Job drawing, mm, ordinate dimensions from the low corner. One solid piece. A direction names the side the tool comes from. Coordinates: 2 decimals unless noted, no trailing zeros. Loops run counter-clockwise (first coordinate to the right, second up) from the corner with the lowest first, then second, coordinate; pieces in that order, holes last. Notation, with made-up numbers: (-18.5, 62.5) -> (7.5, 62.5) arc R13 ccw to (7.5, 80.5) -> close; hole circle Ø4 at (33.5, 89). An arc over 180 degrees is marked (long way). Use one line per item in the form item = value. Start each with the question number.
(1) Band-saw the part on A-A on x = 2.5. Give the cut face in (y, z).
(2) 3-axis set-ups, long thin cutter, end or side, ignore diameter. For the marked faces 1 and 2: which of +Z, -Z, +X, -X, +Y, -Y reach the whole face in a straight line?
(3) Pin check, flat tips, straight feed: P1, Ø2, axis at x = 2, y = 8.5, coming from the -Z side; P2, Ø1.5, axis at y = 5.5, z = 4.5, coming from the -X side; P3, Ø2, axis at y = 10.5, z = 2, coming from the -X side. Stop position of each tip, or through.
(4) Band-saw the part on B-B on z = 2.5. Give the cut face in (x, y), then the cut area to 3 significant figures.
(5) Band-saw the part on D-D on y = 8.25. Give the cut face in (x, z).
(6) Band-saw the part on C-C on x = 1.35. Give the cut face in (y, z), then the cut area to 3 significant figures.
(7) Drill centre lines: L1, parallel to Y at x = 2.5, z = 3.2; L2, parallel to Y at x = 2.35, z = 0.4; L3, parallel to X at y = 8, z = 2.6. Where is each one in solid material? Low to high. Write a range as [from, to].
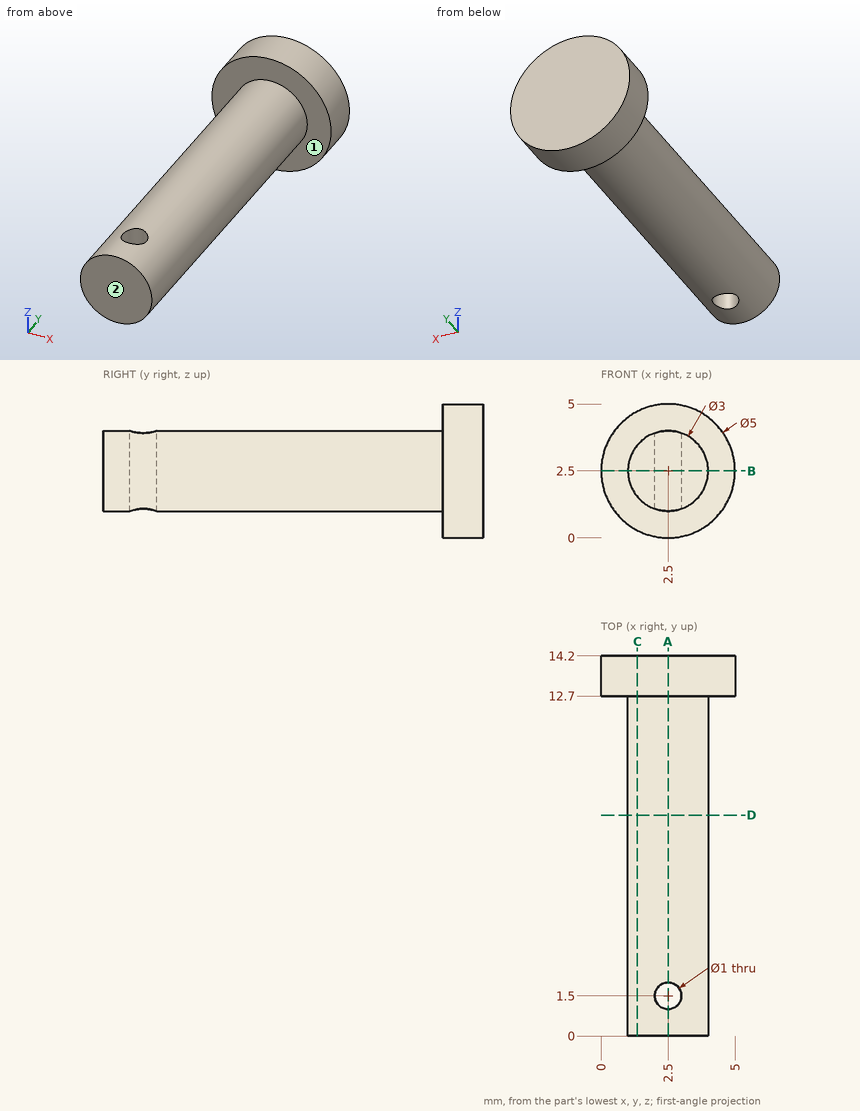
A:
q1.outline = (0, 1) -> (1, 1) -> (1, 4) -> (0, 4) -> close; (2, 1) -> (12.7, 1) -> (12.7, 0) -> (14.2, 0) -> (14.2, 5) -> (12.7, 5) -> (12.7, 4) -> (2, 4) -> close
q2.face_1 = -Y
q2.face_2 = +Z, -Z, +X, -X, -Y
q3.P1 = 1
q3.P2 = 1.67
q3.P3 = 1
q4.outline = (0, 12.7) -> (1, 12.7) -> (1, 0) -> (4, 0) -> (4, 12.7) -> (5, 12.7) -> (5, 14.2) -> (0, 14.2) -> close; hole circle Ø1 at (2.5, 1.5)
q4.area = 44.8 mm²
q5.outline = circle Ø3 at (2.5, 2.5)
q6.outline = (0, 1.54) -> (12.7, 1.54) -> (12.7, 0.28) -> (14.2, 0.28) -> (14.2, 4.72) -> (12.7, 4.72) -> (12.7, 3.46) -> (0, 3.46) -> close
q6.area = 31.1 mm²
q7.L1 = [0, 1], [2, 14.2]
q7.L2 = [12.7, 14.2]
q7.L3 = [1, 4]
